Source: CAD feature listing. Evaluate the final solid. Frame: model axes, mm. Face numbers are marked on the shaded views. Give positions to 0.01 mm unless a question says otherwise; leave off trailing zeros. Loops run counter-clockwise (first coordinate to the right, second up) from the corner with the lowest first, then second, coordinate; pieces in that order, holes last.
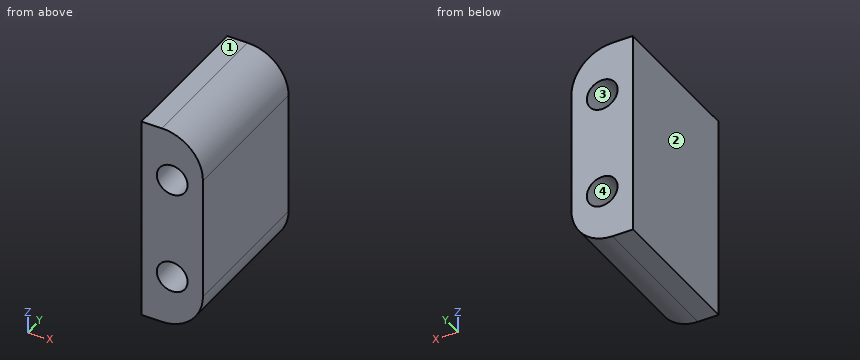
Autodesk Inventor part; units mm, degrees
ref_plane "YZ Plane" through (0, 0, 0) normal (1, 0, 0) x (0, 1, 0)
ref_plane "XZ Plane" through (0, 0, 0) normal (0, 1, 0) x (-1, 0, 0)
ref_plane "XY Plane" through (0, 0, 0) normal (0, 0, 1) x (1, 0, 0)
sketch "Sketch1" plane through (0, 0, 0) normal (1, 0, 0) x (0, 1, 0)
  line L0 (0, 0) -> (14.5, 0)
  line L1 (14.5, 0) -> (14.5, -20)
  line L2 (14.5, -20) -> (0, -20)
  line L3 (0, -20) -> (0, 0)
  dimension "d0" = 14.5
  dimension "d1" = 20
extrude "Extrusion1" add sketch "Sketch1" along normal blind 6
sketch "Sketch2" plane through (0, 14.5, 0) normal (0, 1, 0) x (1, 0, 0)
  line L0 (0, 0) -> (3, 0)
  line L1 (3, 0) -> (3, 5)
  line L2 (3, 5) -> (0, 5)
  line L3 (0, 5) -> (0, 0)
  line L4 (0, 20) -> (6, 20)
  line L5 (6, 20) -> (3, 20)
  line L6 (3, 20) -> (3, 15)
  line L7 (3, 15) -> (6, 15)
  line L8 (6, 15) -> (6, 20)
  circle A0 centre (3, 5) radius 1.5
  circle A1 centre (3, 15) radius 1.5
  dimension "d4" = 3
  dimension "d5" = 5
  dimension "d6" = 3
  dimension "d7" = 5
  dimension "d8" = 3
  dimension "d9" = 3
extrude "Extrusion2" cut sketch "Sketch2" against normal blind 164 contours A0 L2 L1 | L1 L2 A0 | A1 L7 L6 | L6 L7 A1
fillet "Fillet1" radius 4 2 edges at (6, 7.25, 0) (6, 7.25, -20)
properties part number "shoe_lace"
(1) Ray query, line 1 along X through (y, z) = (4, -15); line 2 along Z through (x, y) = (4.05, 12.75); line 3 along Z through (x, y) = (4.2, 4). Return the intervals inside material, ascending.
A:
line 1: x = 0 to 1.5, 4.5 to 6
line 2: z = -19.43 to -16.07, -13.93 to -6.07, -3.93 to -0.57
line 3: z = -19.34 to -15.9, -14.1 to -5.9, -4.1 to -0.66
(2) Section A-A, the plane y = 9.25. Return the cut outline in (x, z), then the cut area to 3 significant figures.
A:
outline: (0, -20) - (2, -20) arc R4 ccw to (6, -16) - (6, -4) arc R4 ccw to (2, 0) - (0, 0) - close; hole circle Ø3 at (3, -15); hole circle Ø3 at (3, -5)
area: 99.0 mm2
(3) Section B-B, the plane z = -5. Return the cut outline in (x, y).
A:
outline: (0, 0) - (1.5, 0) - (1.5, 14.5) - (0, 14.5) - close; (4.5, 0) - (6, 0) - (6, 14.5) - (4.5, 14.5) - close
(4) Mould query, pull axis X, two halves, no side actions, for the marked faces 1, 2, 3 and 4. Classes: pulls with the +X half, pulls with the -X half, needs draft (parallel to the pull), parting line crosses it, or undercut.
A:
face 1: needs draft
face 2: pulls with the -X half
face 3: undercut
face 4: undercut
(5) Section D-D, the plane z = -14. Return the cut outline in (x, y), then the cut area to 3 significant figures.
A:
outline: (0, 0) - (1.88, 0) - (1.88, 14.5) - (0, 14.5) - close; (4.12, 0) - (6, 0) - (6, 14.5) - (4.12, 14.5) - close
area: 54.6 mm2
(6) First-contact query: pin 1 (2 mm diameter, centred on x = 3.5, y = 9, fed in from -Z); pin 2 (2.5 mm diameter, centred on x = 3, z = -5, fed in from -Y). Flat tips, straight axial feed; report the tip coordinate or a pass-through.
A:
pin 1: stops at z = -19.97
pin 2: passes through
(7) Section C-C, the plane x = 3. Return the cut outline in (y, z).
A:
outline: (0, -19.87) - (14.5, -19.87) - (14.5, -16.5) - (0, -16.5) - close; (0, -13.5) - (14.5, -13.5) - (14.5, -6.5) - (0, -6.5) - close; (0, -3.5) - (14.5, -3.5) - (14.5, -0.13) - (0, -0.13) - close
